Can you work these out from the model? Positions are in its coordinate system, mm. A direction names the side the tool comes from. Round coordinates to 2 decimals unless told otherwise and drop trailing zeros. Loops run counter-clockwise (first coordinate to the right, second up) from the corner with the lowest first, then second, coordinate; pieces in that order, holes last.
```python
from build123d import *

# Parameters (mm, degrees)
FILLET1_R          = 2.5
CHAMFER1_SIZE      = 0.5
SKETCH3_R          = 2.25
CUT_EXTRUDE1_DEPTH = 18
CHAMFER2_SIZE      = 1


with BuildPart() as part:
    # Sketch1 → Revolve1 (revolve)
    with BuildSketch(Plane.XY):
        Polygon((4, 22), (4, 20), (1.5, 20), (0, 14), (0, 4), (14, 4), (14, 0), (-3, 0), (-3, 14), (-1, 22), align=None)
    revolve(axis=Axis((0, 0, 0), (1, 0, 0)))

    # Fillet1
    fillet1_edges = [part.edges().sort_by_distance(p)[0] for p in [
        (-1, -22, 0),
        (-3, -14, 0),
        (0, -4, 0),
        (0, -14, 0),
    ]]
    fillet(fillet1_edges, radius=FILLET1_R)

    # Chamfer1
    chamfer1_edges = [part.edges().sort_by_distance(p)[0] for p in [
        (4, -20, 0),
        (14, -4, 0),
    ]]
    chamfer(chamfer1_edges, length=CHAMFER1_SIZE)

    # Sketch3 → Cut-Extrude1 (cut, through all)
    with BuildSketch(Plane.ZY.offset(3)):
        Circle(SKETCH3_R)
    extrude(amount=-CUT_EXTRUDE1_DEPTH, mode=Mode.SUBTRACT)

    # Chamfer2
    chamfer2_edges = [part.edges().sort_by_distance(p)[0] for p in [
        (-3, 0, -2.25),
    ]]
    chamfer(chamfer2_edges, length=CHAMFER2_SIZE)


solid = part.part
```
(1) If I drill on line 1 (Z direction, x = 1.75, y = 11.5) (3 decimals); line 2 (X direction, y = -6.5, z = 7.5); line 3 (Y direction, x = 1.75, z = -7.5), over which ranges is the centre line in solid material (lowest first)?
(2) Suppose I cut it at A-A (x = 11.5). Write out the boundary of the cut face in (y, z), then the cut area to 3 significant figures.
(3) We'd pull the mould along Y, two halves only. Please class faces 1 (the cylindrical face through (2.486, -4.336, -19.524)), 2 (the cylindrical face through (2.5, 20.32, -8.43)), 3 (the flat face through (4, 15, -15)): released by +Y, released by -Y, zero draft, split by the parting line, or undercut.
(4) For pin 1 (2 mm diameter, centred on y = 16, z = -7, fed in from +X); pin 2 (5 mm diameter, centred on x = 1, z = 5, fed in from -Y); pin 3 (1 mm diameter, centred on x = 1.5, z = -7, fed in from +Y), each with a flat end and sliding along its axis, tell me the tip position at first contact or that it passes through.
(5) Which directions (+Z, -Z, +X, -X, +Y, -Y) give clear straight access to the entire face, cutting with the end or side of a thin tool? Please do faces 4 (the cylindrical face through (8.077, -0.867, -3.905)), 5 (the flat face through (14, 2.3, -0.7)).
Check result:
1. line 1: z = -18.755 to -16.363, 16.363 to 18.755
1. line 2: x = -3 to 0
1. line 3: y = -20.68 to -18.54, 18.54 to 20.68
2. outline: circle Ø8 at (0, 0); hole circle Ø4.5 at (0, 0)
2. area: 34.4 mm2
3. face 1: undercut
3. face 2: split by the parting line
3. face 3: zero draft
4. pin 1: stops at x = 1.12
4. pin 2: stops at y = -21.86
4. pin 3: stops at y = 21.02
5. face 4: +X
5. face 5: +Z, -Z, +X, +Y, -Y
